Autodesk Inventor part; units mm, degrees
ref_plane "YZ Plane" through (0, 0, 0) normal (1, 0, 0) x (0, 1, 0)
ref_plane "XZ Plane" through (0, 0, 0) normal (0, 1, 0) x (-1, 0, 0)
ref_plane "XY Plane" through (0, 0, 0) normal (0, 0, 1) x (1, 0, 0)
sketch "Sketch1" plane through (0, 0, 0) normal (0, 1, 0) x (-1, 0, 0)
  line L0 (0, 0) -> (66.03, 0)
  line L1 (66.03, 0) -> (66.03, -23.8)
  line L2 (66.03, -23.8) -> (0, -23.8)
  line L3 (0, -23.8) -> (0, 0)
  dimension "d0" = 66.03
  dimension "d1" = 23.8
extrude "Extrusion1" add sketch "Sketch1" along normal blind 1.0583
sketch "Sketch2" plane through (0, 1.0583, 0) normal (0, 1, 0) x (1, 0, 0)
  line L0 (0, 0) -> (0, 23.8)
  line L1 (-66.03, 0) -> (0, 0)
  point P0 (-60.325, 2.54)
  point P1 (-2.54, 2.54)
  point P2 (-2.54, 20.955)
  point P3 (-60.325, 20.955)
  dimension "d4" = 60.325
  dimension "d5" = 60.325
  dimension "d6" = 2.54
  dimension "d7" = 2.54
  dimension "d8" = 2.54
  dimension "d9" = 2.54
  dimension "d10" = 20.955
  dimension "d11" = 20.955
hole "Hole1" at (-60.325, 1.0583, -2.54) at (-2.54, 1.0583, -2.54) at (-2.54, 1.0583, -20.955) at (-60.325, 1.0583, -20.955) direction (0, -1, 0) diameter 3.81 end through all
properties part number "PCB"
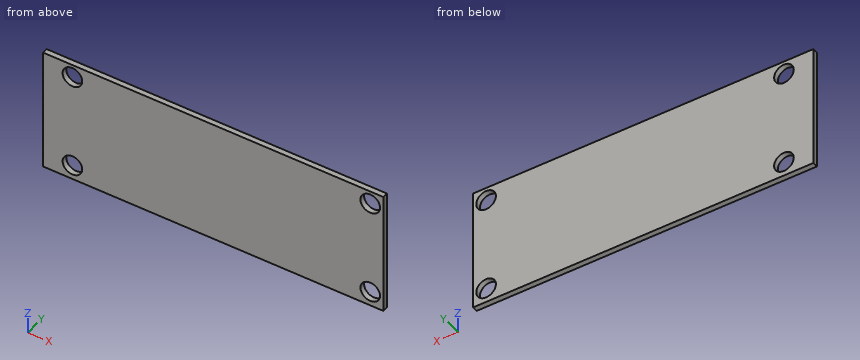
Source: CAD feature listing. Evaluate the final solid. Frame: model axes, mm. Give positions to 0.01 mm unless a question says otherwise; leave off trailing zeros. Loops run counter-clockwise (first coordinate to the right, second up) from the corner with the lowest first, then second, coordinate; pieces in that order, holes last. Notation, with made-up numbers: (-9, 88.25) -> (34, 88.25) arc R18 cw to (34, 104.25) -> close; hole circle Ø3 at (44.5, 3.5). An arc over 180 degrees is marked (long way). Put each result on its own line as item: value. Start each with the question number.
1) Material intervals for probe 1 along X at (y, z) = (0.8, -2.54) (3 decimals); probe 2 along Z at (x, y) = (-2.54, 0.7) (3 decimals); probe 3 along X at (y, z) = (0.7, -20), sorted ascending.
2) Cut plane B-B (z = -2.54). Return loops of the section in (x, y) (3 decimals), then the cut area to 3 significant figures.
3) Cut plane C-C (y = 0.7). Return loops of the section in (x, z) (3 decimals).
4) Cut plane A-A (x = -2.54). Return loops of the section in (y, z) (3 decimals).
Results are:
1. probe 1: x = -66.03 to -62.23, -58.42 to -4.445, -0.635 to 0
1. probe 2: z = -23.8 to -22.86, -19.05 to -4.445, -0.635 to 0
1. probe 3: x = -66.03 to -61.97, -58.68 to -4.19, -0.89 to 0
2. outline: (-66.03, 0) -> (-62.23, 0) -> (-62.23, 1.058) -> (-66.03, 1.058) -> close; (-58.42, 0) -> (-4.445, 0) -> (-4.445, 1.058) -> (-58.42, 1.058) -> close; (-0.635, 0) -> (0, 0) -> (0, 1.058) -> (-0.635, 1.058) -> close
2. area: 61.8 mm2
3. outline: (-66.03, -23.8) -> (0, -23.8) -> (0, 0) -> (-66.03, 0) -> close; hole circle Ø3.81 at (-60.325, -20.955); hole circle Ø3.81 at (-60.325, -2.54); hole circle Ø3.81 at (-2.54, -20.955); hole circle Ø3.81 at (-2.54, -2.54)
4. outline: (0, -23.8) -> (1.058, -23.8) -> (1.058, -22.86) -> (0, -22.86) -> close; (0, -19.05) -> (1.058, -19.05) -> (1.058, -4.445) -> (0, -4.445) -> close; (0, -0.635) -> (1.058, -0.635) -> (1.058, 0) -> (0, 0) -> close
